Source: three-view drawing plus pictorial views. Frame: mm from the lowest corner of the part. Coordinates: 2 decimals unless noted, no trailing zeros. Write each loop counter-clockwise with the first axis right and the second up, starting at its lowest first coordinate (ties: lowest second). Pieces come first, ordered by that corner, then holes. Notation, with made-up numbers: M 34.25,-30 L 49.25,-30 A14 ccw 49.25,-15 Z; hole C 19.5,-21.75 d2. An arc over 180 degrees is marked long. Answer as a JSON object with one key per item and string values. Group by question number.
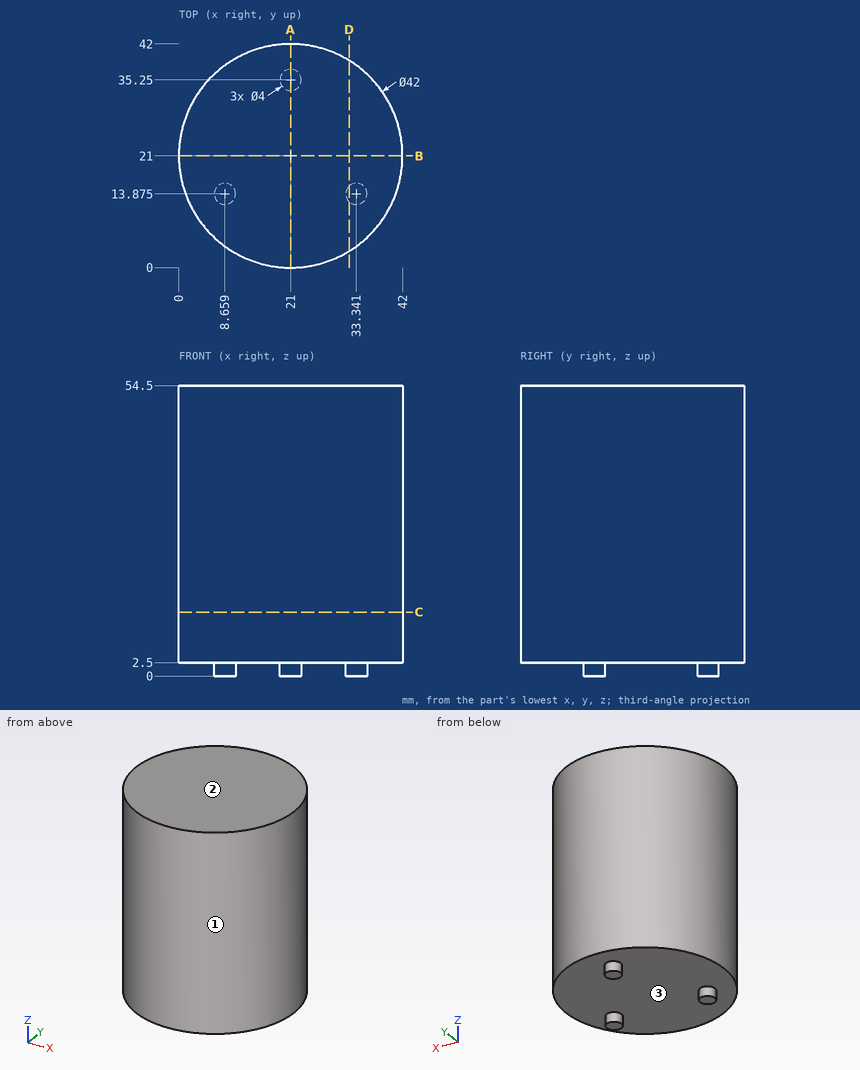
Q1. Line query: line 1 (Z direction, x = 32.5, y = 5.5); line 2 (Y direction, x = 20.5, z = 51.5); line 3 (Y direction, x = 7, z = 47.5). Output: solid intervals per line, ascending. Write a range as from..to.
Q2. Draft query along Z for the marked faces 1, 2 and 3. Return one class per face: released by +Z, released by -Z, zero draft, split by the parting line, or undercut.
Q3. Section A-A, the plane x = 21. Return the cut outline in (y, z), and give its area (3 significant figures).
Q4. Section C-C, the plane z = 12. Return the cut outline in (x, y).
Q5. Section B-B, the plane y = 21. Return the cut outline in (x, z).
Q6. Pin query (flat end, axial travel): pin 1 Ø5 at (x, z) = (6, 49) entering from +Y (1 decimal); pin 2 Ø6 at (x, y) = (26, 17.5) entering from -Z; pin 3 Ø3 at (y, z) = (37, 34.5) entering from +X. Return the tip coordinate at first contact, or that it passes through.
Q7. Section D-D, the plane x = 32. Return the cut outline in (y, z), and give its area (3 significant figures).
Filled in:
{
 "1": {"line 1": "2.5..54.5", "line 2": "0.01..41.99", "line 3": "5.35..36.65"},
 "2": {"face 1": "zero draft", "face 2": "released by +Z", "face 3": "released by -Z"},
 "3": {"outline": "M 0,2.5 L 33.25,2.5 L 33.25,0 L 37.25,0 L 37.25,2.5 L 42,2.5 L 42,54.5 L 0,54.5 Z", "area": "2,190 mm^2"},
 "4": {"outline": "C 21,21 d42"},
 "5": {"outline": "M 0,2.5 L 42,2.5 L 42,54.5 L 0,54.5 Z"},
 "6": {"pin 1": "y = 37.9", "pin 2": "z = 2.5", "pin 3": "x = 36.19"},
 "7": {"outline": "M 3.11,2.5 L 12.39,2.5 L 12.39,0 L 15.36,0 L 15.36,2.5 L 38.89,2.5 L 38.89,54.5 L 3.11,54.5 Z", "area": "1,870 mm^2"}
}
